Part model, mm, in its own coordinate system. Give positions to 0.01 mm unless a question says otherwise; leave off trailing zeros. Order: outer loops, then holes, each group sorted by start corner. A loop starts at its lowest first (then second) coordinate and runs counter-clockwise, first axis right, second up. Notation, with made-up numbers: M 0.5,61 L 10.5,61 A22 ccw 10.5,84 Z; hole C -38,44.5 d2. An arc over 180 degrees is marked long. Answer as a JSON object with one key per item and string values.
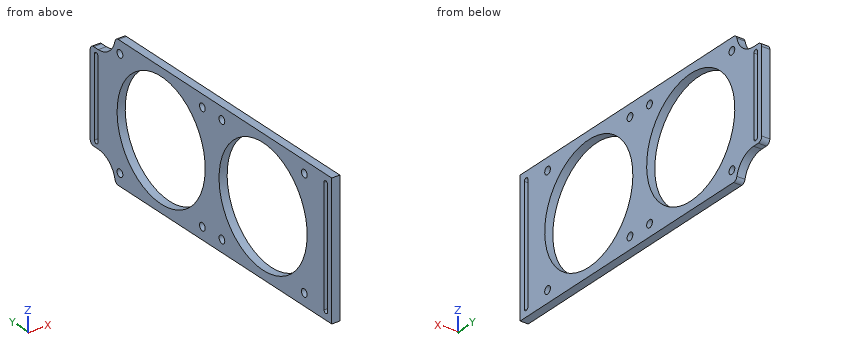
from build123d import *

# Parameters (mm, degrees)
SKETCH2_R                 = 38.5
SKETCH2_W                 = 4
SKETCH2_H                 = 189.008661332
BOSS_EXTRUDE2_DEPTH       = 5.334
F_3_0MM_DOWEL_SLOT1_DEPTH = 5.334
F_3_0MM_DOWEL_SLOT2_DEPTH = 5.334
FILLET1_R                 = 15
FILLET2_R                 = 3
F_5_0MM_DOWEL_HOLE1_D     = 5


# Read off the part's stored shape, not the designer's step: Ø3.0mm Dowel Slot1, Ø3.0mm Dowel Slot2
with BuildPart() as part:
    # Sketch2 → Boss-Extrude2 (new body)
    # profile 1 of 3: a face of its own
    with BuildSketch(Plane(origin=(0, 0, 0), x_dir=(0, 0, -1), z_dir=(1, 0, 0))):
        Polygon((28.490859753, 116.416616863), (28.490859753, 94.390736923), (38.490859753, 94.390736923), (38.490859753, -94.617924409), (-41.509140247, -94.617924409), (-41.509140247, 94.390736923), (-31.509140247, 94.390736923), (-31.509140247, 116.416616863), align=None)
        with Locations((-1.509140247, 54.390736923)):
            Circle(SKETCH2_R, mode=Mode.SUBTRACT)
        with Locations((-1.509140247, -34.676182382)):
            Circle(SKETCH2_R, mode=Mode.SUBTRACT)
    # profile 2 of 3: a face of its own
    with BuildSketch(Plane(origin=(0, 0, 0), x_dir=(0, 0, -1), z_dir=(1, 0, 0))):
        with Locations((-43.509140247, -0.113593743)):
            Rectangle(SKETCH2_W, SKETCH2_H)
    # profile 3 of 3: a face of its own
    with BuildSketch(Plane(origin=(0, 0, 0), x_dir=(0, 0, -1), z_dir=(1, 0, 0))):
        with Locations((40.490859753, -0.113593743)):
            Rectangle(SKETCH2_W, SKETCH2_H)
    extrude(amount=BOSS_EXTRUDE2_DEPTH)

    # Ø3.0mm Dowel Slot1 outline → Ø3.0mm Dowel Slot1 (cut)
    with BuildSketch(Plane.YZ):
        with BuildLine():
            ThreePointArc((-87.91563933, 39.992900247), (-89.41563933, 41.492900247), (-90.91563933, 39.992900247))
            Line((-90.91563933, 39.992900247), (-90.91563933, -37.007099753))
            ThreePointArc((-90.91563933, -37.007099753), (-89.41563933, -38.507099753), (-87.91563933, -37.007099753))
            Line((-87.91563933, -37.007099753), (-87.91563933, 39.992900247))
        make_face()
    extrude(amount=F_3_0MM_DOWEL_SLOT1_DEPTH, mode=Mode.SUBTRACT)

    # Ø3.0mm Dowel Slot2 outline → Ø3.0mm Dowel Slot2 (cut)
    with BuildSketch(Plane.YZ):
        with BuildLine():
            ThreePointArc((112.653676893, 27.509140247), (111.153676893, 29.009140247), (109.653676893, 27.509140247))
            Line((109.653676893, 27.509140247), (109.653676893, -24.490859753))
            ThreePointArc((109.653676893, -24.490859753), (111.153676893, -25.990859753), (112.653676893, -24.490859753))
            Line((112.653676893, -24.490859753), (112.653676893, 27.509140247))
        make_face()
    extrude(amount=F_3_0MM_DOWEL_SLOT2_DEPTH, mode=Mode.SUBTRACT)

    # Fillet1
    # the kernel refuses this fillet: 15 mm, written as the material it adds along each edge
    with BuildSketch(Plane(origin=(0, 94.390736923, 31.509140247), x_dir=(0, 1, 0), z_dir=(1, 0, 0))) as fillet1_piece_1:
        with BuildLine():
            CenterArc((14.966629547, 15), FILLET1_R, 183.822553729, 86.177446271)
            Line((0, 14), (-0.299332591, 13.98))
            ThreePointArc((-0.299332591, 13.98), (-0.3, 7), (-0.3, 0))
            Line((-0.3, 0), (0, -0.3))
            Line((0, -0.3), (14.966629547, -0.3))
            Line((14.966629547, -0.3), (14.966629547, 0))
        make_face()
    extrude(amount=5.334)
    with BuildSketch(Plane(origin=(0, 94.390736923, -28.490859753), x_dir=(0, 1, 0), z_dir=(1, 0, 0))) as fillet1_piece_2:
        with BuildLine():
            CenterArc((14.966629547, -15), FILLET1_R, 90, 86.177446271)
            Line((0, -14), (-0.299332591, -13.98))
            ThreePointArc((-0.299332591, -13.98), (-0.3, -7), (-0.3, 0))
            Line((-0.3, 0), (0, 0.3))
            Line((0, 0.3), (14.966629547, 0.3))
            Line((14.966629547, 0.3), (14.966629547, 0))
        make_face()
    extrude(amount=5.334)

    # Fillet2
    fillet2_edges = [part.edges().sort_by_distance(p)[0] for p in [
        (2.667, 94.390736923, -42.490859753),
        (2.667, 94.390736923, 45.509140247),
        (2.667, 116.416616863, 31.509140247),
        (2.667, 116.416616863, -28.490859753),
    ]]
    fillet(fillet2_edges, radius=FILLET2_R)

    # Ø5.0mm Dowel Hole1 (through all)
    with Locations(Plane.ZY):
        with Locations((-34.490859753, 90.390736923), (37.509140247, 90.390736923), (-34.490859753, 18.390736923), (37.509140247, 18.390736923), (37.509140247, 1.323817618), (-34.490859753, 1.323817618), (-34.490859753, -70.676182382), (37.509140247, -70.676182382)):
            Hole(F_5_0MM_DOWEL_HOLE1_D / 2)


solid = part.part
1. Cut at B-B on z = -9.5. Give the cut face in (x, y).
Worked answers:
{"outline": "M 0,-94.62 L 5.33,-94.62 L 5.33,-90.92 L 0,-90.92 Z; M 0,-87.92 L 5.33,-87.92 L 5.33,-71.57 L 0,-71.57 Z; M 0,2.22 L 5.33,2.22 L 5.33,17.5 L 0,17.5 Z; M 0,91.28 L 5.33,91.28 L 5.33,109.65 L 0,109.65 Z; M 0,112.65 L 5.33,112.65 L 5.33,116.42 L 0,116.42 Z"}
2. Cut at C-C on x = 1.2. State how many separate pieces and enclosed holes the cut face has, plus the area to 3 significant figures.
Worked answers:
{"separate pieces": "1", "enclosed holes": "12", "area": "8,170 mm^2"}
3. Cut at A-A on y = 38. Give the cut face in (x, z).
Worked answers:
{"outline": "M 0,-42.49 L 5.33,-42.49 L 5.33,-33.33 L 0,-33.33 Z; M 0,36.35 L 5.33,36.35 L 5.33,45.51 L 0,45.51 Z"}
4. Cut at D-D on y = 67.5. Give the cut face in (x, z), plus the area to 3 significant figures.
Worked answers:
{"outline": "M 0,-42.49 L 5.33,-42.49 L 5.33,-34.69 L 0,-34.69 Z; M 0,37.71 L 5.33,37.71 L 5.33,45.51 L 0,45.51 Z", "area": "83.2 mm^2"}
5. Probe line 1 along Y through (x, z) = (5.05, 25); line 2 along Y through (x, z) = (5.15, 21.5); line 3 along Y through (x, z) = (2, -27.5). List the from-to ranges inside material, lowest first.
Worked answers:
{"line 1": "y = -94.62 to -90.92, -87.92 to -65.18, -4.17 to 23.89, 84.89 to 109.65, 112.65 to 116.42", "line 2": "y = -94.62 to -90.92, -87.92 to -67.58, -1.77 to 21.49, 87.29 to 109.65, 112.65 to 116.42", "line 3": "y = -94.62 to -90.92, -87.92 to -59.99, -9.36 to 29.08, 79.7 to 115.64"}
6. Pin check, flat tips, straight feed: P1, Ø4.5, axis at y = 1.32, z = 37.51, coming from the +X side; P2, Ø3, axis at x = 3, y = 111.5, coming from the -Z side; P3, Ø2, axis at x = 3.5, y = 110.5, coming from the +Z side. Stop position of each tip, or through.
Worked answers:
{"P1": "passes through", "P2": "stops at z = -28.49", "P3": "stops at z = 31.51"}
